Source: CAD feature listing. Evaluate the final solid. Frame: model axes, mm. Face numbers are marked on the shaded views. A direction names the side the tool comes from. Give positions to 0.01 mm unless a question says otherwise; leave off trailing zeros. Loops run counter-clockwise (first coordinate to the right, second up) from the corner with the lowest first, then second, coordinate; pieces in that order, holes last.
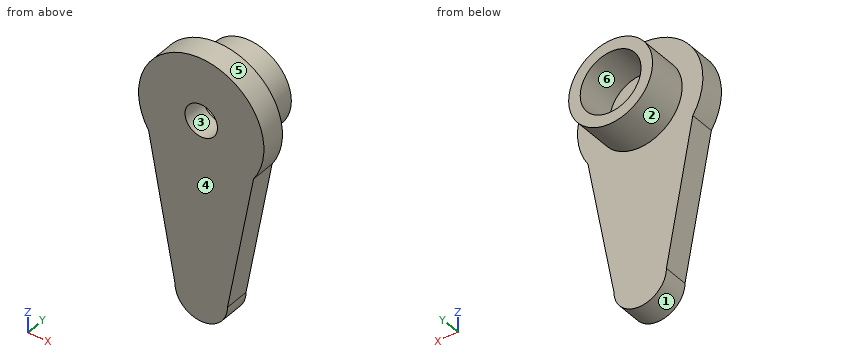
```python
from build123d import *

# Parameters (mm, degrees)
SKETCH1_R           = 1.55
BOSS_EXTRUDE1_DEPTH = 2.35
SKETCH1_3_R         = 4
SKETCH1_3_R_2       = 2.9
BOSS_EXTRUDE2_DEPTH = 6.1


with BuildPart() as part:
    # Sketch1 → Boss-Extrude1 (new body)
    with BuildSketch(Plane(origin=(0, 0, 0), x_dir=(1, 0, 0), z_dir=(0, 1, 0))):
        with BuildLine():
            Line((-2.5, 16.75), (-5.015451004, 3.247441489))
            ThreePointArc((-5.015451004, 3.247441489), (0.028324767, -5.974932862), (4.984436631, 3.294846957))
            Line((4.984436631, 3.294846957), (2.5, 16.75))
            ThreePointArc((2.5, 16.75), (0, 19.25), (-2.5, 16.75))
        make_face()
        Circle(SKETCH1_R, mode=Mode.SUBTRACT)
    extrude(amount=BOSS_EXTRUDE1_DEPTH)

    # Sketch1<3> → Boss-Extrude2 (add)
    with BuildSketch(Plane(origin=(0, 0, 0), x_dir=(1, 0, 0), z_dir=(0, 1, 0))):
        Circle(SKETCH1_3_R)
        Circle(SKETCH1_3_R_2, mode=Mode.SUBTRACT)
    extrude(amount=BOSS_EXTRUDE2_DEPTH)


solid = part.part
```
(1) Mould query, pull axis X, two halves, no side actions, for the marked faces 3, 4, 5 and 6. Classes: pulls with the +X half, pulls with the -X half, needs draft (parallel to the pull), parting line crosses it, or undercut.
A:
face 3: undercut
face 4: needs draft
face 5: parting line crosses it
face 6: undercut
(2) Section C-C, the plane y = 3.5. Return the cut outline in (x, z), then the cut area to 3 significant figures.
A:
outline: circle Ø8 at (0, 0); hole circle Ø5.8 at (0, 0)
area: 23.8 mm2
(3) Reachability of the marked faces 1 and 2 from +Z, -Z, +X, -X, +Y, -Y: full face, straight path, thin tool, end or side. Return the list, or none.
A:
face 1: -Z, +Y, -Y
face 2: +Y
(4) Section D-D, the plane x = -2.25. Return the cut outline in (y, z).
A:
outline: (0, -17.84) - (2.35, -17.84) - (2.35, -3.31) - (6.1, -3.31) - (6.1, -1.83) - (2.35, -1.83) - (2.35, 1.83) - (6.1, 1.83) - (6.1, 3.31) - (2.35, 3.31) - (2.35, 5.54) - (0, 5.54) - close
(5) Ray query, line 1 along Z through (x, y) = (0, 1.05) (3 decimals); line 2 along Z through (x, y) = (0, 5.2); line 3 along Y through (x, z) = (0.25, -17). Return the intervals inside material, ascending.
A:
line 1: z = -19.25 to -1.55, 1.55 to 5.975
line 2: z = -4 to -2.9, 2.9 to 4
line 3: y = 0 to 2.35
(6) Section B-B, the plane x = 0. Return the cut outline in (y, z) (3 decimals).
A:
outline: (0, -19.25) - (2.35, -19.25) - (2.35, -4) - (6.1, -4) - (6.1, -2.9) - (2.35, -2.9) - (2.35, -1.55) - (0, -1.55) - close; (0, 1.55) - (2.35, 1.55) - (2.35, 2.9) - (6.1, 2.9) - (6.1, 4) - (2.35, 4) - (2.35, 5.975) - (0, 5.975) - close
(7) First-contact query: pin 1 (4 mm diameter, centred on x = 2.5, z = 0.5, fed in from -Y); pin 2 (4.5 mm diameter, centred on x = 0, z = 0.5, fed in from +Y). Flat tips, straight axial feed; report the tip coordinate or a pass-through.
A:
pin 1: stops at y = 0
pin 2: stops at y = 2.35
(8) Section A-A, the plane z = 0. Return the cut outline in (x, y) (3 decimals), then the cut area to 3 significant figures.
A:
outline: (-5.975, 0) - (-1.55, 0) - (-1.55, 2.35) - (-2.9, 2.35) - (-2.9, 6.1) - (-4, 6.1) - (-4, 2.35) - (-5.975, 2.35) - close; (1.55, 0) - (5.975, 0) - (5.975, 2.35) - (4, 2.35) - (4, 6.1) - (2.9, 6.1) - (2.9, 2.35) - (1.55, 2.35) - close
area: 29.0 mm2
